Verification items for the finished model (mm, model axes). Face numbers are marked on the shaded views. A direction names the side the tool comes from. Round coordinates to 2 decimals unless told otherwise and drop trailing zeros. Loops run counter-clockwise (first coordinate to the right, second up) from the corner with the lowest first, then second, coordinate; pieces in that order, holes last. Notation, with made-up numbers: (53.5, -29) -> (99.5, -29) arc R13 ccw to (99.5, -17) -> close; hole circle Ø5 at (-36.5, 12.5). An arc over 180 degrees is marked (long way). Write item = value, one per line.
```python
from build123d import *

# Parameters (mm, degrees)
SKETCH1_W                              = 42.3
SKETCH1_H                              = 42.3
BOSS_EXTRUDE1_DEPTH                    = 6.35
SKETCH2_R                              = 11
SKETCH2_R_2                            = 1.5
CUT_EXTRUDE1_DEPTH                     = 6.35
SKETCH3_W                              = 42.3
SKETCH3_H                              = 6.35
BOSS_EXTRUDE2_DEPTH                    = 12.7
SKETCH4_W                              = 6.35
SKETCH4_H                              = 42.3
BOSS_EXTRUDE3_DEPTH                    = 50
FILLET1_R                              = 6.35
FILLET2_R                              = 6.35
TAP_DRILL_FOR_M8_HELICOIL1_D           = 8.25
TAP_DRILL_FOR_M8_HELICOIL1_DEPTH       = 6.35
TAP_DRILL_FOR_M8_HELICOIL1_CSINK_D     = 8.3
TAP_DRILL_FOR_M8_HELICOIL1_CSINK_ANGLE = 90
FILLET1_OF_MIRROR4_R                   = 6.35
FILLET2_OF_MIRROR4_R                   = 6.35


with BuildPart() as part:
    # Sketch1 → Boss-Extrude1 (new body)
    with BuildSketch(Plane(origin=(0, 0, 0), x_dir=(1, 0, 0), z_dir=(0, 1, 0))):
        with Locations((21.15, -21.15)):
            Rectangle(SKETCH1_W, SKETCH1_H)
    extrude(amount=BOSS_EXTRUDE1_DEPTH)

    # Sketch2 → Cut-Extrude1 (cut)
    with BuildSketch(Plane(origin=(0, 6.35, 0), x_dir=(1, 0, 0), z_dir=(0, 1, 0))):
        with Locations(Location((21.15, -21.15, 0), (0, 0, 270))):
            Circle(SKETCH2_R)
        with Locations(Location((5.65, -5.65, 0), (0, 0, 270))):
            Circle(SKETCH2_R_2)
        with Locations(Location((5.65, -36.65, 0), (0, 0, 270))):
            Circle(SKETCH2_R_2)
        with Locations(Location((36.65, -5.65, 0), (0, 0, 270))):
            Circle(SKETCH2_R_2)
        with Locations(Location((36.65, -36.65, 0), (0, 0, 270))):
            Circle(SKETCH2_R_2)
    extrude(amount=-CUT_EXTRUDE1_DEPTH, mode=Mode.SUBTRACT)

    # Sketch3 → Boss-Extrude2 (add)
    with BuildSketch(Plane(origin=(42.3, 0, 0), x_dir=(0, 0, -1), z_dir=(1, 0, 0))):
        with Locations((-21.15, 3.175)):
            Rectangle(SKETCH3_W, SKETCH3_H)
    boss_extrude2 = extrude(amount=BOSS_EXTRUDE2_DEPTH)

    # Sketch4 → Boss-Extrude3 (add)
    with BuildSketch(Plane(origin=(0, 6.35, 0), x_dir=(1, 0, 0), z_dir=(0, 1, 0))):
        with Locations((51.825, -21.15)):
            Rectangle(SKETCH4_W, SKETCH4_H)
    boss_extrude3 = extrude(amount=BOSS_EXTRUDE3_DEPTH)

    # Fillet1
    fillet1_edges = [part.edges().sort_by_distance(p)[0] for p in [
        (48.65, 6.35, 21.15),
    ]]
    fillet(fillet1_edges, radius=FILLET1_R)

    # Fillet2
    fillet2_edges = [part.edges().sort_by_distance(p)[0] for p in [
        (55, 0, 21.15),
    ]]
    fillet(fillet2_edges, radius=FILLET2_R)

    # Tap Drill for M8 Helicoil1
    with Locations(Plane.ZY.offset(-48.65)):
        with Locations((21.15, 44.35), (21.15, 28.35)):
            tap_drill_for_m8_helicoil1 = CounterSinkHole(TAP_DRILL_FOR_M8_HELICOIL1_D / 2, TAP_DRILL_FOR_M8_HELICOIL1_CSINK_D / 2, depth=TAP_DRILL_FOR_M8_HELICOIL1_DEPTH, counter_sink_angle=TAP_DRILL_FOR_M8_HELICOIL1_CSINK_ANGLE)

    # Mirror4: Boss-Extrude2, Boss-Extrude3, Tap Drill for M8 Helicoil1 across plane
    add(boss_extrude2.mirror(Plane.ZY.offset(-21.15)))
    add(boss_extrude3.mirror(Plane.ZY.offset(-21.15)))
    add(tap_drill_for_m8_helicoil1.mirror(Plane.ZY.offset(-21.15)), mode=Mode.SUBTRACT)

    # Fillet1 of Mirror4
    fillet1_of_mirror4_edges = [part.edges().sort_by_distance(p)[0] for p in [
        (-6.35, 6.35, 21.15),
    ]]
    fillet(fillet1_of_mirror4_edges, radius=FILLET1_OF_MIRROR4_R)

    # Fillet2 of Mirror4
    fillet2_of_mirror4_edges = [part.edges().sort_by_distance(p)[0] for p in [
        (-12.7, 0, 21.15),
    ]]
    fillet(fillet2_of_mirror4_edges, radius=FILLET2_OF_MIRROR4_R)


solid = part.part
```
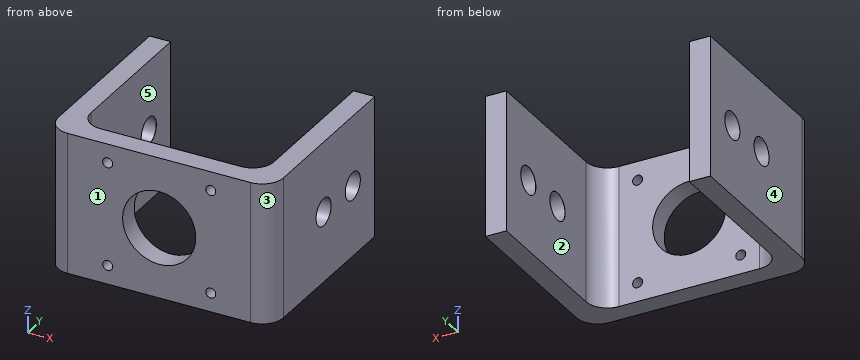
(1) Sectioned sample at A-A, the plane x = 5.65. Record the cut outline in (y, z), and give its area (3 significant figures).
Filled sheet:
outline = (0, 0) -> (6.35, 0) -> (6.35, 4.15) -> (0, 4.15) -> close; (0, 7.15) -> (6.35, 7.15) -> (6.35, 35.15) -> (0, 35.15) -> close; (0, 38.15) -> (6.35, 38.15) -> (6.35, 42.3) -> (0, 42.3) -> close
area = 231 mm2
(2) Sectioned sample at C-C, the plane y = 28.35. Record the cut outline in (x, z) (3 decimals).
Filled sheet:
outline = (-12.7, 0) -> (-6.35, 0) -> (-6.35, 17) -> (-6.375, 17.025) -> (-12.7, 17.025) -> close; (-12.7, 25.275) -> (-6.375, 25.275) -> (-6.35, 25.3) -> (-6.35, 42.3) -> (-12.7, 42.3) -> close; (48.65, 0) -> (55, 0) -> (55, 17.025) -> (48.675, 17.025) -> (48.65, 17) -> close; (48.65, 25.3) -> (48.675, 25.275) -> (55, 25.275) -> (55, 42.3) -> (48.65, 42.3) -> close
(3) Set-up check for the marked faces 1 and 2: record each of +Z, -Z, +X, -X, +Y, -Y from which the full face is reachable in a straight line by a thin tool's end or side.
Filled sheet:
face_1 = +Z, -Z, +X, -X, -Y
face_2 = +Z, -Z, +Y
(4) Go/stop test with flat-tipped pins: pin 1 Ø3.5 at (x, z) = (5.65, 36.65) entering from +Y; pin 2 Ø10.5 at (y, z) = (44.35, 21.15) entering from +X; pin 3 Ø10 at (x, z) = (3.5, 17) entering from +Y. Record where each tip stops, or that it passes through.
Filled sheet:
pin_1 = 6.35
pin_2 = 55
pin_3 = 6.53
(5) Sectioned sample at B-B, the plane y = 21.5. Record the cut outline in (x, z), and give its area (3 significant figures).
Filled sheet:
outline = (-12.7, 0) -> (-6.35, 0) -> (-6.35, 42.3) -> (-12.7, 42.3) -> close; (48.65, 0) -> (55, 0) -> (55, 42.3) -> (48.65, 42.3) -> close
area = 537 mm2
(6) Draft check along X on the marked faces 3, 4 and 5. Enter one of: released by +X, released by -X, zero draft, split by the parting line, or undercut.
Filled sheet:
face_3 = released by +X
face_4 = released by -X
face_5 = undercut
(7) Sectioned sample at D-D, the plane z = 5.65. Record the cut outline in (x, y), and give its area (3 significant figures).
Filled sheet:
outline = (-12.7, 6.35) arc R6.35 ccw to (-6.35, 0) -> (4.15, 0) -> (4.15, 6.35) -> (0, 6.35) arc R6.35 cw to (-6.35, 12.7) -> (-6.35, 56.35) -> (-12.7, 56.35) -> close; (7.15, 0) -> (35.15, 0) -> (35.15, 6.35) -> (7.15, 6.35) -> close; (38.15, 0) -> (48.65, 0) arc R6.35 ccw to (55, 6.35) -> (55, 56.35) -> (48.65, 56.35) -> (48.65, 12.7) arc R6.35 cw to (42.3, 6.35) -> (38.15, 6.35) -> close
area = 1,030 mm2
(8) Material ranges on probe 1 along X at (y, z) = (23, 37); probe 2 along X at (y, z) = (3, 5), recorded low to high. Write a range as from..to.
Filled sheet:
probe_1 = -12.7..-6.35, 48.65..55
probe_2 = -11.74..4.3, 7..35.3, 38..54.04
